Drawing for the job (mm, zero at the part's lowest x, y, z). Give positions to 0.01 mm unless a question says otherwise; leave off trailing zeros. Order: outer loops, then holes, each group sorted by start corner. A loop starts at its lowest first (then second) coordinate and runs counter-clockwise, first axis right, second up. Notation, with made-up numbers: (-38.75, 78.5) -> (20.25, 78.5) arc R30 cw to (20.25, 101.5) -> close; hole circle Ø5 at (-33.5, 13.25). An arc over 180 degrees is marked (long way). One line per item, written item: value. Start each with the question number.
(1) Saw through at A-A on z = 70. Give the cut face in (x, y) (1 decimal).
(2) Saw through at B-B on y = 19.5. Give the cut face in (x, z) (1 decimal), plus the area to 3 significant figures.
(3) Saw through at C-C on z = 84. Give the cut face in (x, y) (1 decimal), plus the area to 3 significant figures.
(4) Probe line 1 (Z direction, x = 103.5, y = 71.5) (1 decimal); line 2 (Z direction, x = 86, y = 167); line 3 (X direction, y = 131.5, z = 73) (1 decimal). List the from-to ranges inside material, lowest first.
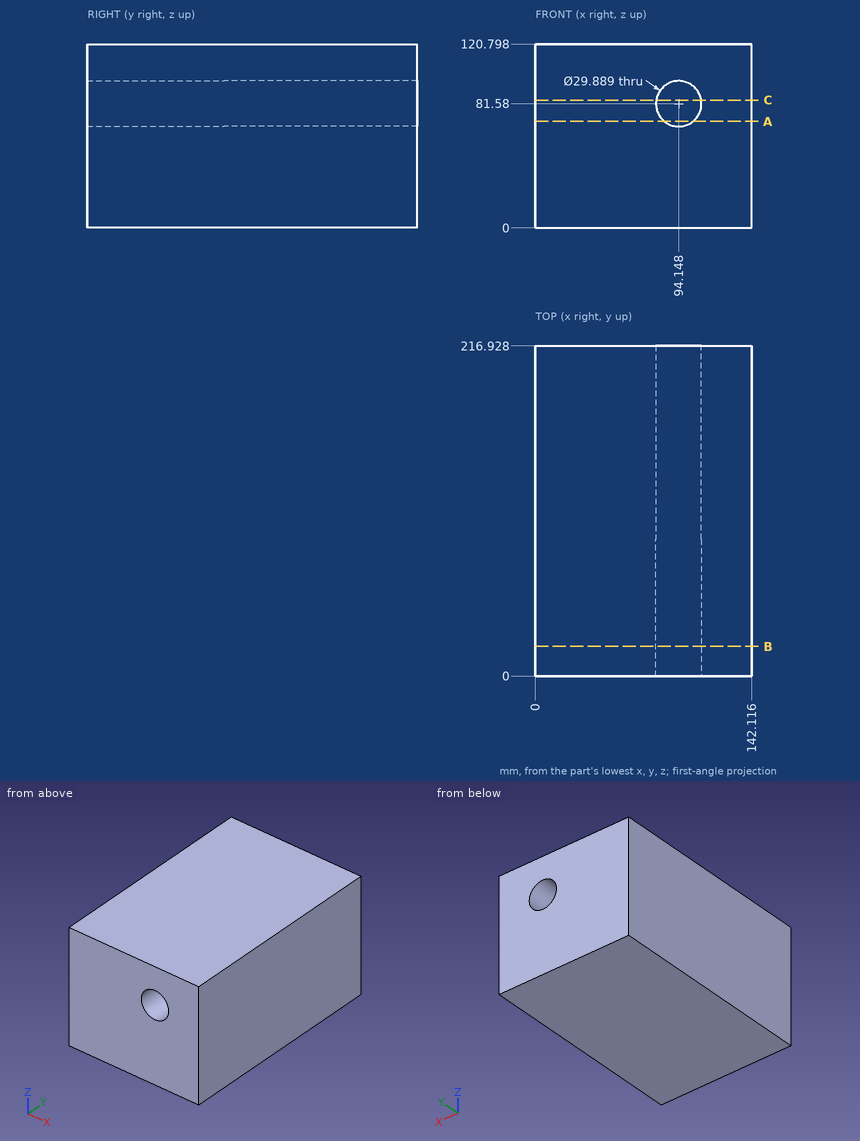
Results below:
1. outline: (0, 0) -> (84.7, 0) -> (84.7, 216.9) -> (0, 216.9) -> close; (103.6, 0) -> (142.1, 0) -> (142.1, 216.9) -> (103.6, 216.9) -> close
2. outline: (0, 0) -> (142.1, 0) -> (142.1, 120.8) -> (0, 120.8) -> close; hole circle Ø29.9 at (94.1, 81.6)
2. area: 16,500 mm²
3. outline: (0, 0) -> (79.4, 0) -> (79.4, 216.9) -> (0, 216.9) -> close; (108.9, 0) -> (142.1, 0) -> (142.1, 216.9) -> (108.9, 216.9) -> close
3. area: 24,400 mm²
4. line 1: z = 0 to 69.9, 93.2 to 120.8
4. line 2: z = 0 to 69.05, 94.11 to 120.8
4. line 3: x = 0 to 81.9, 106.4 to 142.1
